The listing builds one solid part. Answer for the finished solid, in the listing's coordinates (mm). Face numbers are marked on the shaded views. A direction names the side the tool comes from. Round coordinates to 2 decimals unless told otherwise and drop trailing zeros. Write each loop counter-clockwise with the first axis right and the second up, starting at its lowest first coordinate (ties: lowest second). Pieces come first, ordered by that corner, then holes. Notation, with made-up numbers: (65.5, 62) - (121.5, 62) arc R32 ccw to (121.5, 88) - close; hole circle Ø11 at (32, 22). An arc over 180 degrees is marked (long way). Answer in a Markdown table with one row per item.
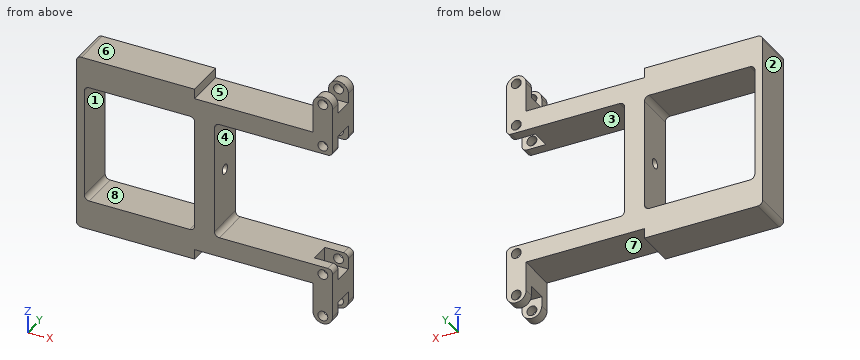
from build123d import *

# Parameters (mm, degrees)
SKETCH1_W           = 60
SKETCH1_H           = 90
BOSS_EXTRUDE1_DEPTH = 20
EXTRUDE_THIN2_DEPTH = 20
SKETCH4_W           = 52
SKETCH4_H           = 60
CUT_EXTRUDE1_DEPTH  = 20
SKETCH5_W           = 4
SKETCH5_H           = 60
CUT_EXTRUDE2_DEPTH  = 20
SKETCH6_R           = 2.5
CUT_EXTRUDE5_DEPTH  = 20
SKETCH8_R           = 2.5
CUT_EXTRUDE6_DEPTH  = 20
FILLET1_R           = 2.5
SKETCH10_R          = 2.5
CUT_EXTRUDE8_DEPTH  = 20
FILLET4_RADIUS      = 5
FILLET4_LENGTH      = 20
FILLET5_RADIUS      = 5
FILLET5_LENGTH      = 20
FILLET7_R           = 2.5
SKETCH14_W          = 10
SKETCH14_H          = 10
SKETCH14_W_2        = 12
SKETCH14_H_2        = 8
CUT_EXTRUDE12_DEPTH = 5


with BuildPart() as part:
    # Sketch1 → Boss-Extrude1 (new body)
    with BuildSketch(Plane(origin=(0, 0, 0), x_dir=(1, 0, 0), z_dir=(0, 1, 0))):
        Rectangle(SKETCH1_W, SKETCH1_H)
    extrude(amount=BOSS_EXTRUDE1_DEPTH)

    # Sketch2 → Extrude-Thin2 (add)
    with BuildSketch(Plane(origin=(0, 20, 0), x_dir=(1, 0, 0), z_dir=(0, 1, 0))):
        Polygon((90, -60), (90, -40), (30, -40), (30, 0), (30, 40), (90, 40), (90, 60), (100, 60), (100, 30), (40, 30), (40, 0), (40, -30), (100, -30), (100, -60), align=None)
    extrude(amount=-EXTRUDE_THIN2_DEPTH)

    # Sketch4 → Cut-Extrude1 (cut)
    with BuildSketch(Plane(origin=(0, 20, 0), x_dir=(1, 0, 0), z_dir=(0, 1, 0))):
        Rectangle(SKETCH4_W, SKETCH4_H)
    extrude(amount=-CUT_EXTRUDE1_DEPTH, mode=Mode.SUBTRACT)

    # Sketch5 → Cut-Extrude2 (cut)
    with BuildSketch(Plane(origin=(0, 20, 0), x_dir=(1, 0, 0), z_dir=(0, 1, 0))):
        with Locations((28, 0)):
            Rectangle(SKETCH5_W, SKETCH5_H)
    extrude(amount=-CUT_EXTRUDE2_DEPTH, mode=Mode.SUBTRACT)

    # Sketch6 → Cut-Extrude5 (cut, symmetric)
    with BuildSketch(Plane(origin=(0, 10, 0), x_dir=(1, 0, 0), z_dir=(0, 1, 0))):
        with Locations(Location((95, -34, 0), (0, 0, 270))):
            Circle(SKETCH6_R)
    cut_extrude5 = extrude(amount=CUT_EXTRUDE5_DEPTH, both=True, mode=Mode.SUBTRACT)

    # Sketch8 → Cut-Extrude6 (cut, symmetric)
    with BuildSketch(Plane(origin=(0, 10, 0), x_dir=(1, 0, 0), z_dir=(0, 1, 0))):
        with Locations(Location((95, -56, 0), (0, 0, 270))):
            Circle(SKETCH8_R)
    cut_extrude6 = extrude(amount=CUT_EXTRUDE6_DEPTH, both=True, mode=Mode.SUBTRACT)

    # Mirror1: Cut-Extrude5, Cut-Extrude6 across plane
    add(cut_extrude5.mirror(Plane.XY), mode=Mode.SUBTRACT)
    add(cut_extrude6.mirror(Plane.XY), mode=Mode.SUBTRACT)

    # Fillet1
    fillet1_edges = [part.edges().sort_by_distance(p)[0] for p in [
        (40, 10, -30),
        (40, 10, 30),
        (-26, 10, 30),
        (-26, 10, -30),
        (30, 10, -30),
        (30, 10, 30),
        (-30, 10, -45),
        (-30, 10, 45),
    ]]
    fillet(fillet1_edges, radius=FILLET1_R)

    # Sketch10 → Cut-Extrude8 (cut)
    with BuildSketch(Plane(origin=(40, 0, 0), x_dir=(0, 0, -1), z_dir=(1, 0, 0))):
        with Locations((0, 10)):
            Circle(SKETCH10_R)
    extrude(amount=-CUT_EXTRUDE8_DEPTH, mode=Mode.SUBTRACT)

    # Fillet4: full round fillet: the end face becomes a half cylinder, R = half its width
    fillet4_face = Plane((95, 10, 60), x_dir=(0, 1, 0), z_dir=(0, 0, 1))  # on the end face: x along it, z out of the body
    fillet4_slab = fillet4_face.offset(-FILLET4_RADIUS / 2) * Box(FILLET4_LENGTH, 2 * FILLET4_RADIUS, FILLET4_RADIUS, mode=Mode.PRIVATE)  # the body's end, R deep
    fillet4_round = Plane((95, 10, 55), x_dir=(0, 0, 1), z_dir=(0, 1, 0)) * Cylinder(FILLET4_RADIUS, FILLET4_LENGTH, mode=Mode.PRIVATE)  # its axis R under the face
    add(fillet4_slab - fillet4_round, mode=Mode.SUBTRACT)

    # Fillet5: full round fillet: the end face becomes a half cylinder, R = half its width
    fillet5_face = Plane((95, 10, -60), x_dir=(0, -1, 0), z_dir=(0, 0, -1))  # on the end face: x along it, z out of the body
    fillet5_slab = fillet5_face.offset(-FILLET5_RADIUS / 2) * Box(FILLET5_LENGTH, 2 * FILLET5_RADIUS, FILLET5_RADIUS, mode=Mode.PRIVATE)  # the body's end, R deep
    fillet5_round = Plane((95, 10, -55), x_dir=(0, 0, -1), z_dir=(0, -1, 0)) * Cylinder(FILLET5_RADIUS, FILLET5_LENGTH, mode=Mode.PRIVATE)  # its axis R under the face
    add(fillet5_slab - fillet5_round, mode=Mode.SUBTRACT)

    # Fillet7
    fillet7_edges = [part.edges().sort_by_distance(p)[0] for p in [
        (100, 10, -30),
        (100, 10, 30),
    ]]
    fillet(fillet7_edges, radius=FILLET7_R)

    # Sketch14 → Cut-Extrude12 (cut, symmetric)
    with BuildSketch(Plane(origin=(0, 10, 0), x_dir=(1, 0, 0), z_dir=(0, 1, 0))):
        with Locations((95, 55)):
            Rectangle(SKETCH14_W, SKETCH14_H)
        with Locations((94, 34)):
            Rectangle(SKETCH14_W_2, SKETCH14_H_2)
    cut_extrude12 = extrude(amount=CUT_EXTRUDE12_DEPTH, both=True, mode=Mode.SUBTRACT)

    # Mirror3: Cut-Extrude12 across plane
    add(cut_extrude12.mirror(Plane.XY), mode=Mode.SUBTRACT)


solid = part.part
(1) Section C-C (z = 18) is taken. Give the vertices of the cut face in (x, y), and give its area (3 significant figures).
Checked values:
| item | result |
|---|---|
| outline | (-30, 0) - (-26, 0) - (-26, 20) - (-30, 20) - close; (30, 0) - (40, 0) - (40, 20) - (30, 20) - close |
| area | 280 mm2 |
(2) Section D-D (x = 95) is taken. State how many separate pieces and enclosed holes the cut face has, and give its area (3 significant figures).
Checked values:
| item | result |
|---|---|
| separate pieces | 10 |
| enclosed holes | 0 |
| area | 640 mm2 |
(3) Find the intervals of material crossed by line 1 (X direction, y = 16.25, z = 34); line 2 (Z direction, x = 1.5, y = 7); line 3 (Z direction, x = 94.5, y = 6.75), in increasing order.
Checked values:
| item | result |
|---|---|
| line 1 | x = -30 to 92.5, 97.5 to 100 |
| line 2 | z = -45 to -30, 30 to 45 |
| line 3 | z = -50 to -38, 38 to 50 |
(4) For a pull along X with two mould halves and no side action, classify the marked faces 1, 2 and 3 as pulls with the +X half, pulls with the -X half, needs draft (parallel to the pull), parting line crosses it, or undercut.
Checked values:
| item | result |
|---|---|
| face 1 | undercut |
| face 2 | pulls with the -X half |
| face 3 | needs draft |
(5) For the marked faces 4, 5, 6, 7 and 8, determine the directions among +Z, -Z, +X, -X, +Y, -Y from which every point of the face is accessible in a straight line to the end or side of a thin tool.
Checked values:
| item | result |
|---|---|
| face 4 | +X, +Y, -Y |
| face 5 | +Z, +Y, -Y |
| face 6 | +Z, -X, +Y, -Y |
| face 7 | -Z, +Y, -Y |
| face 8 | +Y, -Y |
(6) Section A-A (x = 68.5) is taken. Give the vertices of the cut face in (y, z).
Checked values:
| item | result |
|---|---|
| outline | (0, -40) - (20, -40) - (20, -30) - (0, -30) - close; (0, 30) - (20, 30) - (20, 40) - (0, 40) - close |
(7) Section B-B (z = 0) is taken. Give the vertices of the cut face in (x, y).
Checked values:
| item | result |
|---|---|
| outline | (-30, 0) - (-26, 0) - (-26, 20) - (-30, 20) - close; (30, 0) - (40, 0) - (40, 7.5) - (30, 7.5) - close; (30, 12.5) - (40, 12.5) - (40, 20) - (30, 20) - close |
(8) Flat-ended cylindrical pins translate along their axes: pin 1 (12 mm diameter, centred on y = 17, z = -5.5, fed in from +X); pin 2 (5 mm diameter, centred on x = 97, y = 10, fed in from +Z); pin 3 (1.5 mm diameter, centred on x = 3, y = 13.5, fed in from -Z); pin 4 (4.5 mm diameter, centred on x = 95, z = 34, fed in from -Y). Find the tip coordinate at first contact, or state that the pin passes through.
Checked values:
| item | result |
|---|---|
| pin 1 | stops at x = 40 |
| pin 2 | stops at z = 50 |
| pin 3 | stops at z = -45 |
| pin 4 | passes through |
